Could you check a few things on this model? Use its own coordinates, in mm. Give positions to 0.01 mm unless a question says otherwise; leave off trailing zeros. Loops run counter-clockwise (first coordinate to the right, second up) from the corner with the lowest first, then second, coordinate; pieces in that order, holes last. Notation, with made-up numbers: (-23, 54.5) - (31, 54.5) arc R15 cw to (31, 81.5) - close; hole circle Ø8 at (89, 20). An arc over 180 degrees is marked (long way). One line per item, written item: value. Start each with the question number.
Q1. If I drill on line 1 (Z direction, x = 0.4, y = -0.5); line 2 (Y direction, x = -0.15, z = 25.4); line 3 (Y direction, x = -0.3, z = 127.5), over which ranges is the centre line in solid material (lowest first)? Write a range as from..to.
Q2. I'm going to push a flat-ended pin straight in: P1, Ø5, axis at y = 0, z = 127, coming from the -X side. Where does the tip first touch, or does it pass through?
Q3. If we mould it in two halves opening along Z, with no side actions, what happens to faces 1 (the face through (-0.007, 0.49, 26.957)), 2 (the face through (-0.01, 0.07, 74.57)), 3 (the face through (-0.508, 2, 75))? For each: released by +Z, released by -Z, zero draft, split by the parting line, or undercut.
Q4. I want a section at D-D (z = 96.5). Please give me the cut outline in (x, y).
Q5. I want a section at C-C (x = 0.15). Please give me the cut outline in (y, z).
Q6. I want a section at A-A (z = 25.4). Please give me the cut outline in (x, y).
Q7. I want a section at B-B (y = 0). Please give me the cut outline in (x, z), then the cut area to 3 significant figures.
```python
from build123d import *

# Parameters (mm, degrees)
BOSS_EXTRUDE3_DEPTH       = 152.4
F_4_CLEARANCE_HOLE2_D     = 3.2639
F_4_CLEARANCE_HOLE2_DEPTH = 1.524
F_4_CLEARANCE_HOLE2_TIP   = 0.980574487


with BuildPart() as part:
    # Sketch2 → Boss-Extrude3 (new body)
    with BuildSketch(Plane.XY):
        with BuildLine():
            Line((-0.508, -4.915254952), (-0.508, 6.746875))
            Line((-0.508, 6.746875), (0.508, 6.746875))
            Line((0.508, 6.746875), (0.508, -6.746875))
            ThreePointArc((0.508, -6.746875), (0.236990731, -5.699606171), (-0.508, -4.915254952))
        make_face()
    extrude(amount=BOSS_EXTRUDE3_DEPTH)

    # #4 Clearance Hole2
    with Locations(Plane(origin=(0.508, 0, 0), x_dir=(0, 0, -1), z_dir=(1, 0, 0))):
        with Locations((-25.4, 0), (-76.2, 0), (-177.8, 0), (-127, 0), (-228.6, 0), (-279.4, 0)):
            Hole(F_4_CLEARANCE_HOLE2_D / 2, depth=F_4_CLEARANCE_HOLE2_DEPTH)
            with Locations((0, 0, -(F_4_CLEARANCE_HOLE2_DEPTH + F_4_CLEARANCE_HOLE2_TIP / 2))):  # 118° drill point
                Cone(0, F_4_CLEARANCE_HOLE2_D / 2, F_4_CLEARANCE_HOLE2_TIP, mode=Mode.SUBTRACT)


solid = part.part
```
Worked answers:
1. line 1: z = 0..23.85, 26.95..74.65, 77.75..125.45, 128.55..152.4
1. line 2: y = -5.2..-1.63, 1.63..6.75
1. line 3: y = -5.06..-1.55, 1.55..6.75
2. P1: stops at x = -0.51
3. face 1: undercut
3. face 2: undercut
3. face 3: zero draft
4. outline: (-0.51, -4.92) arc R2.16 cw to (0.51, -6.75) - (0.51, 6.75) - (-0.51, 6.75) - close
5. outline: (-5.56, 0) - (6.75, 0) - (6.75, 152.4) - (-5.56, 152.4) - close; hole circle Ø3.26 at (0, 25.4); hole circle Ø3.26 at (0, 76.2); hole circle Ø3.26 at (0, 127)
6. outline: (-0.51, -4.92) arc R2.16 cw to (0.51, -6.75) - (0.51, -1.63) - (-0.51, -1.63) - close; (-0.51, 1.63) - (0.51, 1.63) - (0.51, 6.75) - (-0.51, 6.75) - close
7. outline: (-0.51, 0) - (0.51, 0) - (0.51, 23.77) - (-0.51, 23.77) - close; (-0.51, 27.03) - (0.51, 27.03) - (0.51, 74.57) - (-0.51, 74.57) - close; (-0.51, 77.83) - (0.51, 77.83) - (0.51, 125.37) - (-0.51, 125.37) - close; (-0.51, 128.63) - (0.51, 128.63) - (0.51, 152.4) - (-0.51, 152.4) - close
7. area: 145 mm²
